Geometry: final body of the model. Coordinates: model frame, mm. A direction names the side the tool comes from. Give positions to 0.01 mm unless a question says otherwise; leave off trailing zeros. Order: outer loops, then holes, each group sorted by start corner. A loop starts at its lowest first (then second) coordinate and runs counter-clockwise, first axis right, second up. Notation, with made-up numbers: M 19,2 L 37,2 A28 cw 37,29 Z; hole C 46.25,83 d11. An arc over 180 degrees is marked long. Use CSV: the item, a comma, the result in double quotes.
```python
from build123d import *

# Parameters (mm, degrees)
SKETCH1_W            = 40
SKETCH1_H            = 40
BOSS_EXTRUDE1_DEPTH  = 2
EXTRUDE_THIN1_START  = 2
SKETCH1_3_W          = 14
SKETCH1_3_H          = 1
EXTRUDE_THIN1_DEPTH  = 11.2
SKETCH3_R            = 1.65
CUT_EXTRUDE1_DEPTH   = 13.2
LPATTERN1_COUNT      = 2
LPATTERN1_PITCH      = 32
LPATTERN1_COUNT_DIR2 = 2
LPATTERN1_PITCH_DIR2 = 32


with BuildPart() as part:
    # Sketch1 → Boss-Extrude1 (new body)
    with BuildSketch(Plane.XY):
        with Locations((21, 22.483732861)):
            Rectangle(SKETCH1_W, SKETCH1_H)
    extrude(amount=BOSS_EXTRUDE1_DEPTH)

    # Sketch1<3> → Extrude-Thin1 (add)
    with BuildSketch(Plane.XY.offset(EXTRUDE_THIN1_START)):
        with Locations((34, 8.699522335)):
            Rectangle(SKETCH1_3_W, SKETCH1_3_H)
        with Locations((34, 11.415311808)):
            Rectangle(SKETCH1_3_W, SKETCH1_3_H)
        with Locations((34, 14.131101282)):
            Rectangle(SKETCH1_3_W, SKETCH1_3_H)
        with Locations((34, 17.752153914)):
            Rectangle(SKETCH1_3_W, SKETCH1_3_H)
        with Locations((34, 20.467943387)):
            Rectangle(SKETCH1_3_W, SKETCH1_3_H)
        with Locations((34, 23.183732861)):
            Rectangle(SKETCH1_3_W, SKETCH1_3_H)
        with Locations((34, 25.899522335)):
            Rectangle(SKETCH1_3_W, SKETCH1_3_H)
        with Locations((34, 29.520574966)):
            Rectangle(SKETCH1_3_W, SKETCH1_3_H)
        with Locations((34, 32.23636444)):
            Rectangle(SKETCH1_3_W, SKETCH1_3_H)
        with Locations((8, 8.699522335)):
            Rectangle(SKETCH1_3_W, SKETCH1_3_H)
        with Locations((8, 11.415311808)):
            Rectangle(SKETCH1_3_W, SKETCH1_3_H)
        with Locations((8, 14.131101282)):
            Rectangle(SKETCH1_3_W, SKETCH1_3_H)
        with Locations((8, 17.752153914)):
            Rectangle(SKETCH1_3_W, SKETCH1_3_H)
        with Locations((8, 20.467943387)):
            Rectangle(SKETCH1_3_W, SKETCH1_3_H)
        with Locations((8, 23.183732861)):
            Rectangle(SKETCH1_3_W, SKETCH1_3_H)
        with Locations((8, 25.899522335)):
            Rectangle(SKETCH1_3_W, SKETCH1_3_H)
        with Locations((8, 29.520574966)):
            Rectangle(SKETCH1_3_W, SKETCH1_3_H)
        with Locations((8, 32.23636444)):
            Rectangle(SKETCH1_3_W, SKETCH1_3_H)
    extrude(amount=EXTRUDE_THIN1_DEPTH)

    # Sketch3 → Cut-Extrude1 (cut)
    with BuildSketch(Plane(origin=(0, 0, 0), x_dir=(-1, 0, 0), z_dir=(0, 0, -1))):
        with Locations((-37, 6.483732861)):
            Circle(SKETCH3_R)
    cut_extrude1 = extrude(amount=-CUT_EXTRUDE1_DEPTH, mode=Mode.SUBTRACT)

    # LPattern1: Cut-Extrude1 2 × 2
    with Locations(*[(-i * LPATTERN1_PITCH, j * LPATTERN1_PITCH_DIR2, 0) for i in range(LPATTERN1_COUNT) for j in range(LPATTERN1_COUNT_DIR2) if (i, j) != (0, 0)]):
        add(cut_extrude1, mode=Mode.SUBTRACT)


solid = part.part
```
1. Line query: line 1 (Y direction, x = 5, z = 0.75); line 2 (X direction, y = 20, z = 3.25); line 3 (Z direction, x = 15.5, y = 36). Output: solid intervals per line, ascending.
Answer:
line 1,"2.48 to 4.83, 8.13 to 36.83, 40.13 to 42.48"
line 2,"1 to 15, 27 to 41"
line 3,"0 to 2"
2. Pin query (flat end, axial travel): pin 1 Ø1 at (x, z) = (11, 12) entering from +Y; pin 2 Ø2.5 at (x, y) = (37, 38.48) entering from -Z; pin 3 Ø5 at (x, z) = (32.5, 8) entering from -Y. Return the tip coordinate at first contact, or that it passes through.
Answer:
pin 1,"y = 32.74"
pin 2,"through"
pin 3,"y = 8.2"
3. Section D-D, the plane y = 27. Return the cut outline in (x, z).
Answer:
outline,"M 1,0 L 41,0 L 41,2 L 1,2 Z"
4. Section B-B, the plane z = 1. Return the cut outline in (x, y).
Answer:
outline,"M 1,2.48 L 41,2.48 L 41,42.48 L 1,42.48 Z; hole C 5,6.48 d3.3; hole C 5,38.48 d3.3; hole C 37,6.48 d3.3; hole C 37,38.48 d3.3"
5. Reachability of faces 1 (the face through (8, 10.915, 8)), 2 (the face through (15, 32, 8)), 3 (the face through (21, 23, 0)) from +Z, -Z, +X, -X, +Y, -Y: full face, straight path, thin tool, end or side. Return the list, or none.
Answer:
face 1,"+Z, +X, -X"
face 2,"+Z, +Y, -Y"
face 3,"-Z, +X, -X, +Y, -Y"
6. Pull-direction query (X, two-part tool) for faces 4 (the face through (8, 14.631, 8)), 5 (the face through (15, 23, 8)); classes: +X half, -X half, draft (parallel to the pull), parting line (faces both ways), or undercut.
Answer:
face 4,"draft"
face 5,"undercut"
7. Section A-A, the plane x = 5. Give the number of separate pieces and of enclosed holes in the cut face, plus the area to 3 significant figures.
Answer:
separate pieces,"3"
enclosed holes,"0"
area,"168 mm2"
